```python
from build123d import *

# Parameters (mm, degrees)
F0_R     = 3.175
F0_R_2   = 3.5
F1_DEPTH = 9


with BuildPart() as f1:
    # F0 (on Top) → F1 (new body)
    with BuildSketch(Plane.XY):
        with BuildLine():
            Line((0, 25.675), (0, 37.5))
            Line((0, 37.5), (-31, 37.5))
            ThreePointArc((-31, 37.5), (-37.363961, 34.863961), (-40, 28.5))
            Line((-40, 28.5), (-40, 27.5))
            ThreePointArc((-40, 27.5), (-44.100505, 17.600505), (-54, 13.5))
            ThreePointArc((-54, 13.5), (-54.707107, 13.207107), (-55, 12.5))
            Line((-55, 12.5), (-55, 0))
            Line((-55, 0), (-46.25, 0))
            ThreePointArc((-46.25, 0), (-41, 5.25), (-35.75, 0))
            Line((-35.75, 0), (-25.675, 0))
            ThreePointArc((-25.675, 0), (-22.5, 3.175), (-19.325, 0))
            Line((-19.325, 0), (-11.5, 0))
            ThreePointArc((-11.5, 0), (-8.131728, 8.131728), (0, 11.5))
            Line((0, 11.5), (0, 19.325))
            ThreePointArc((0, 19.325), (-3.175, 22.5), (0, 25.675))
        make_face()
        with Locations((-26.324893, 26)):
            Circle(F0_R, mode=Mode.SUBTRACT)
        with BuildLine():
            Line((31, 37.5), (0, 37.5))
            Line((0, 37.5), (0, 25.675))
            ThreePointArc((0, 25.675), (2.245064, 24.745064), (3.175, 22.5))
            ThreePointArc((3.175, 22.5), (2.245064, 20.254936), (0, 19.325))
            Line((0, 19.325), (0, 11.5))
            ThreePointArc((0, 11.5), (8.131728, 8.131728), (11.5, 0))
            Line((11.5, 0), (19.325, 0))
            ThreePointArc((19.325, 0), (22.5, 3.175), (25.675, 0))
            Line((25.675, 0), (35.75, 0))
            ThreePointArc((35.75, 0), (41, 5.25), (46.25, 0))
            Line((46.25, 0), (55, 0))
            Line((55, 0), (55, 12.5))
            ThreePointArc((55, 12.5), (54.707107, 13.207107), (54, 13.5))
            ThreePointArc((54, 13.5), (44.100505, 17.600505), (40, 27.5))
            Line((40, 27.5), (40, 28.5))
            ThreePointArc((40, 28.5), (37.363961, 34.863961), (31, 37.5))
        make_face()
        with Locations((26.324893, 26)):
            Circle(F0_R, mode=Mode.SUBTRACT)
        with BuildLine():
            Line((19.325, 0), (11.5, 0))
            ThreePointArc((11.5, 0), (8.131728, -8.131728), (0, -11.5))
            Line((0, -11.5), (0, -19.325))
            ThreePointArc((0, -19.325), (2.245064, -20.254936), (3.175, -22.5))
            ThreePointArc((3.175, -22.5), (2.245064, -24.745064), (0, -25.675))
            Line((0, -25.675), (0, -37.5))
            Line((0, -37.5), (31, -37.5))
            ThreePointArc((31, -37.5), (37.363961, -34.863961), (40, -28.5))
            Line((40, -28.5), (40, -27.5))
            ThreePointArc((40, -27.5), (44.100505, -17.600505), (54, -13.5))
            ThreePointArc((54, -13.5), (54.707107, -13.207107), (55, -12.5))
            Line((55, -12.5), (55, 0))
            Line((55, 0), (46.25, 0))
            ThreePointArc((46.25, 0), (41, -5.25), (35.75, 0))
            Line((35.75, 0), (25.675, 0))
            ThreePointArc((25.675, 0), (22.5, -3.175), (19.325, 0))
        make_face()
        with Locations((26.324893, -26)):
            Circle(F0_R, mode=Mode.SUBTRACT)
        with Locations((35, -11)):
            Circle(F0_R_2, mode=Mode.SUBTRACT)
        with BuildLine():
            ThreePointArc((0, -11.5), (-8.131728, -8.131728), (-11.5, 0))
            Line((-11.5, 0), (-19.325, 0))
            ThreePointArc((-19.325, 0), (-22.5, -3.175), (-25.675, 0))
            Line((-25.675, 0), (-35.75, 0))
            ThreePointArc((-35.75, 0), (-41, -5.25), (-46.25, 0))
            Line((-46.25, 0), (-55, 0))
            Line((-55, 0), (-55, -12.5))
            ThreePointArc((-55, -12.5), (-54.707107, -13.207107), (-54, -13.5))
            ThreePointArc((-54, -13.5), (-44.100505, -17.600505), (-40, -27.5))
            Line((-40, -27.5), (-40, -28.5))
            ThreePointArc((-40, -28.5), (-37.363961, -34.863961), (-31, -37.5))
            Line((-31, -37.5), (0, -37.5))
            Line((0, -37.5), (0, -25.675))
            ThreePointArc((0, -25.675), (-3.175, -22.5), (0, -19.325))
            Line((0, -19.325), (0, -11.5))
        make_face()
        with Locations((-26.324893, -26)):
            Circle(F0_R, mode=Mode.SUBTRACT)
    extrude(amount=F1_DEPTH)


solid = f1.part
```
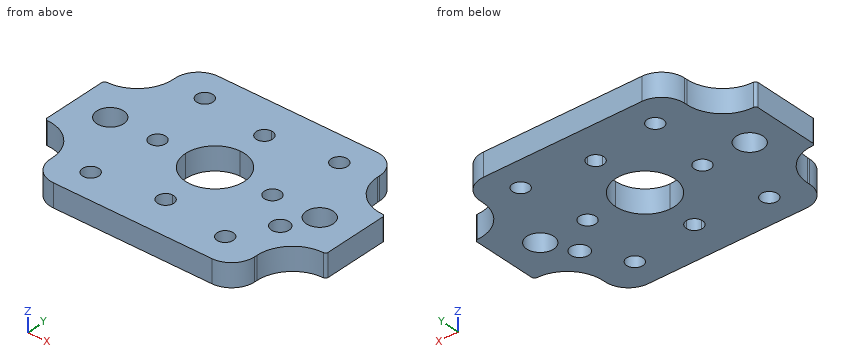
Check sheet for the modelled part. Datum: model origin and axes. Units: mm. Round coordinates to 2 decimals unless told otherwise and drop trailing zeros. Loops run counter-clockwise (first coordinate to the right, second up) from the corner with the lowest first, then second, coordinate; pieces in that order, holes last. Notation, with made-up numbers: (5, -0.75) - (20, -0.75) arc R20 ccw to (20, 8.25) - close; hole circle Ø8 at (76.25, 25). An arc over 180 degrees is marked (long way). Answer as a JSON object with one key per item and string values. Group by question number.
Q1. Gauge pin test, flat ends, axial feed: P1, Ø4, axis at y = 23, z = 3, coming from the +X side; P2, Ø1.1, axis at y = -28, z = 5, coming from the +X side; P3, Ø1.1, axis at y = 28, z = 2.5, coming from the -X side. Record the tip position at first contact, or that the pin passes through.
Q2. Sectioned sample at A-A, the plane y = -9. Enter the section's corners in (x, z).
Q3. Sectioned sample at C-C, the plane z = 7.75. Count the separate pieces of the cut face and the enclosed holes in it, plus the area to 3 significant figures.
Q4. Sectioned sample at B-B, the plane x = 43. Enter the section's corners in (y, z), plus the area to 3 significant figures.
Q5. Sectioned sample at D-D, the plane x = -43.5. Enter the section's corners in (y, z).
Q6. Scan lines: line 1 along Y through (x, z) = (-1.5, 8.25); line 2 along Y through (x, z) = (-22.5, 5.25) (3 decimals); line 3 along X through (y, z) = (-1.5, 4). Record each from-to range of solid material in increasing order. Write a range as [from, to].
Solution:
{
 "1": {"P1": "stops at x = 41.6", "P2": "stops at x = 40", "P3": "stops at x = -40"},
 "2": {"outline": "(-55, 0) - (-7.16, 0) - (-7.16, 9) - (-55, 9) - close; (7.16, 0) - (32.13, 0) - (32.13, 9) - (7.16, 9) - close; (37.87, 0) - (55, 0) - (55, 9) - (37.87, 9) - close"},
 "3": {"separate pieces": "1", "enclosed holes": "12", "area": "6,030 mm²"},
 "4": {"outline": "(-18.84, 0) - (-4.85, 0) - (-4.85, 9) - (-18.84, 9) - close; (4.85, 0) - (18.84, 0) - (18.84, 9) - (4.85, 9) - close", "area": "252 mm²"},
 "5": {"outline": "(-18.24, 0) - (-4.62, 0) - (-4.62, 9) - (-18.24, 9) - close; (4.62, 0) - (18.24, 0) - (18.24, 9) - (4.62, 9) - close"},
 "6": {"line 1": "y = [-37.5, -25.3], [-19.7, -11.4], [11.4, 19.7], [25.3, 37.5]", "line 2": "y = [-37.5, -3.175], [3.175, 37.5]", "line 3": "x = [-55, -46.03], [-35.97, -25.3], [-19.7, -11.4], [11.4, 19.7], [25.3, 35.97], [46.03, 55]"}
}
